The model under review builds one solid part; all positions refer to its coordinate system, in mm. A direction names the side the tool comes from. Give positions to 0.01 mm unless a question says otherwise; leave off trailing zeros. Write item = value, one per line. Start each with the question number.
1. For faces 1 (the face through (0, -15, -91)), 2 (the face through (2, -29, -130)), list the 3-axis set-ups (+Z, -Z, +X, -X, +Y, -Y) from which the entire face can be reached by the end or side of a thin tool; tool diameter is ignored.
2. For pin 1 (3 mm diameter, centred on x = 1, z = -40.5, fed in from -Y); pin 2 (2.5 mm diameter, centred on x = 3, y = -29.5, fed in from -Z); pin 3 (1.5 mm diameter, centred on x = 4, y = -24, fed in from +Z), all flat-tipped, find the tip position at first contact; note any pin that passes through.
3. Wall thickness on line 1 along Y through (x, z) = (3.65, -27); line 2 along Y through (x, z) = (0.6, -81); line 3 along Z through (x, y) = (0.55, -17.5): over which ranges is each line inside the solid? List them lowest first. Write a range as from..to.
from build123d import *

# Parameters (mm, degrees)
EXTRUDE_1_DEPTH = 5
FILLET_6_R      = 5
FILLET_7_R      = 2
FILLET_8_R      = 5


# Read off the part's stored shape, not the designer's step: 凸台-拉伸1
with BuildPart() as part:
    # 凸台-拉伸1 outline → 凸台-拉伸1 (new body)
    with BuildSketch(Plane(origin=(0, 0, 0), x_dir=(0, 0, -1), z_dir=(1, 0, 0))):
        with BuildLine():
            add(Edge.make_bspline(
                [(0, -14.903846424), (2.951295662, -4.14849373), (13.496276672, -1.883966721), (29.52909514, 0), (83.401333812, 0)],
                knots=[0, 0, 0, 0, 0, 1, 1, 1, 1, 1], degree=4))
            add(Edge.make_bspline(
                [(0, -14.903846424), (7.045609734, -22.926953025), (13.86614676, -26.583220196), (29.227640995, -32.621761678), (74.300319088, -39.100169059), (130, -39.92714285)],
                knots=[0, 0, 0, 0, 0, 0, 0.966542999, 0.966542999, 0.966542999, 0.966542999, 0.966542999, 0.966542999], degree=5))
            Line((130, -39.92714285), (130, -20))
            add(Edge.make_bspline(
                [(130, -20), (142.554964398, -11.053747082), (149.196912904, -34.934175524), (158.630756241, -5.373255264), (163.289648635, -33.936740498), (166.072200522, -10.144868391), (180, -20)],
                knots=[0, 0, 0, 0, 0, 0, 0, 1, 1, 1, 1, 1, 1, 1], degree=6))
            Line((180, -20), (180, 0))
            Line((180, 0), (83.401333812, 0))
        make_face()
    extrude(amount=EXTRUDE_1_DEPTH)

    # 圆角6
    fillet_6_edges = [part.edges().sort_by_distance(p)[0] for p in [
        (2.5, -20, -130),
    ]]
    fillet(fillet_6_edges, radius=FILLET_6_R)

    # 圆角7
    fillet_7_edges = [part.edges().sort_by_distance(p)[0] for p in [
        (2.5, -20, -180),
    ]]
    fillet(fillet_7_edges, radius=FILLET_7_R)

    # 圆角8
    fillet_8_edges = [part.edges().sort_by_distance(p)[0] for p in [
        (2.5, 0, -180),
        (2.5, -39.92714285, -130),
    ]]
    fillet(fillet_8_edges, radius=FILLET_8_R)


solid = part.part
Final values:
q1.face_1 = +Z, -Z, -X, +Y, -Y
q1.face_2 = -Z, +X, -X, -Y
q2.pin_1 = -32.34
q2.pin_2 = -130
q2.pin_3 = -10.53
q3.line_1 = -29.11..-1.59
q3.line_2 = -37.4..0
q3.line_3 = -179.79..-2.47
